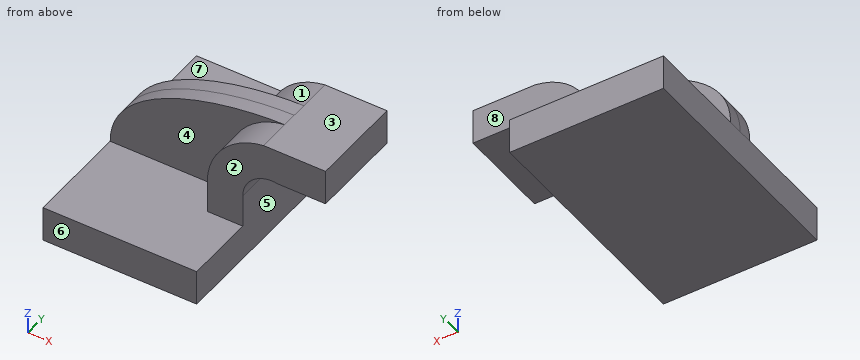
from build123d import *

# Parameters (mm, degrees)
F1_DEPTH = 63.5
F0_W     = 25.4
F0_H     = 19.05
F2_DEPTH = 25.4
F3_DEPTH = 7.9375


with BuildPart() as f1:
    # F0 (on Front) → F1 (new body, symmetric)
    with BuildSketch(Plane.XZ):
        Polygon((41.275, -9.525), (41.275, 9.525), (22.225, 9.525), (-41.275, 9.525), (-41.275, -9.525), align=None)
    extrude(amount=F1_DEPTH, both=True)

    # F0 (on Front) → F2 (join, symmetric)
    with BuildSketch(Plane.XZ):
        with BuildLine():
            Line((22.225, 9.525), (41.275, 9.525))
            Line((41.275, 9.525), (41.275, 27.32094))
            ThreePointArc((41.275, 27.32094), (47.109768, 39.617662), (60.325, 42.8752))
            Line((60.325, 42.8752), (60.325, 61.9252))
            Line((60.325, 61.9252), (52.427625, 61.9252))
            ThreePointArc((52.427625, 61.9252), (30.837602, 50.286422), (22.225, 27.32094))
            Line((22.225, 27.32094), (22.225, 9.525))
        make_face()
        with Locations((73.025, 52.4002)):
            Rectangle(F0_W, F0_H)
    extrude(amount=F2_DEPTH, both=True)

    # F0 (on Front) → F3 (join, symmetric)
    with BuildSketch(Plane.XZ):
        with BuildLine():
            Line((-41.275, 9.525), (22.225, 9.525))
            Line((22.225, 9.525), (22.225, 27.32094))
            ThreePointArc((22.225, 27.32094), (30.837602, 50.286422), (52.427625, 61.9252))
            add(Edge.make_bspline(
                [(-41.275, 9.525), (-41.49317, 47.016986), (14.679759, 61.308946), (52.427625, 61.9252)],
                knots=[0, 0, 0, 0, 107.359037, 107.359037, 107.359037, 107.359037], degree=3))
        make_face()
    extrude(amount=F3_DEPTH, both=True)


solid = f1.part
CAD build for the part. Positions are in the model's coordinates, mm. Face numbers are marked on the shaded views. A direction names the side the tool comes from. Round coordinates to 2 decimals unless told otherwise and drop trailing zeros. Loops run counter-clockwise (first coordinate to the right, second up) from the corner with the lowest first, then second, coordinate; pieces in that order, holes last. Notation, with made-up numbers: (53.25, -25.5) - (81.25, -25.5) arc R29 ccw to (81.25, 1.5) - close; hole circle Ø9 at (60.25, 31). An arc over 180 degrees is marked (long way). Put each result on its own line as item: value.
1. Slice it at A-A on y = -10.5. List the corners of the cut face in (x, z) (3 decimals).
Geometry check:
outline: (-41.275, -9.525) - (41.275, -9.525) - (41.275, 27.321) arc R15.875 cw to (60.325, 42.875) - (85.725, 42.875) - (85.725, 61.925) - (52.428, 61.925) arc R34.925 ccw to (22.225, 27.321) - (22.225, 9.525) - (-41.275, 9.525) - close
2. Two-plate mould, pull along Y, no slides. Class the marked faces 6, 7 and 8: released by +Y, released by -Y, zero draft, split by the parting line, or undercut.
Geometry check:
face 6: released by -Y
face 7: zero draft
face 8: released by +Y
3. Pin check, flat tips, straight feed: P1, Ø12.5, axis at x = 72.5, y = -7.5, coming from the -Z side; P2, Ø19, axis at y = -17.5, z = 21.5, coming from the -X side (3 decimals); P3, Ø1.5, axis at x = 20.5, z = 11, coming from the +Y side. Stop position of each tip, or through.
Geometry check:
P1: z = 42.88
P2: x = 22.225
P3: y = 7.94
4. Slice it at C-C on z = 5. List the corners of the cut face in (x, y) (3 decimals).
Geometry check:
outline: (-41.275, -63.5) - (41.275, -63.5) - (41.275, 63.5) - (-41.275, 63.5) - close
5. Slice it at B-B on x = 75.5. List the corners of the cut face in (y, z).
Geometry check:
outline: (-25.4, 42.88) - (25.4, 42.88) - (25.4, 61.93) - (-25.4, 61.93) - close
6. Wall check: line 1 (Z direction, x = 65, y = 4.5); line 2 (Y direction, x = 40.5, z = 53); line 3 (Y direction, x = 2, z = 28.5). Give the ranges that are in metal, low to high.
Geometry check:
line 1: 42.88 to 61.93
line 2: -25.4 to 25.4
line 3: -7.94 to 7.94
7. 3-axis set-ups, long thin cutter, end or side, ignore diameter. For the marked faces 1, 2, 3, 4 and 5: which of +Z, -Z, +X, -X, +Y, -Y reach the whole face in a straight line?
Geometry check:
face 1: +Z, -X, +Y
face 2: +Z, +X, -X, -Y
face 3: +Z, +X, -X, +Y, -Y
face 4: +Z, -X, -Y
face 5: -Z, +X, +Y, -Y
